```python
from build123d import *

# Parameters (mm, degrees)
SKETCH_1_W      = 68.5
SKETCH_1_H      = 36.5
SKETCH_1_W_2    = 56.5
SKETCH_1_H_2    = 24.5
EXTRUDE_1_DEPTH = 1
FILLET_1_R      = 3


with BuildPart() as part:
    # 草图1 → 凸台-拉伸1 (new body)
    with BuildSketch(Plane(origin=(0, 0, 0), x_dir=(1, 0, 0), z_dir=(0, 1, 0))):
        with Locations((-124.87745098, 48.691176471)):
            Rectangle(SKETCH_1_W, SKETCH_1_H)
        with Locations((-124.87745098, 48.691176471)):
            Rectangle(SKETCH_1_W_2, SKETCH_1_H_2, mode=Mode.SUBTRACT)
    extrude(amount=EXTRUDE_1_DEPTH)

    # 圆角1
    fillet_1_edges = [part.edges().sort_by_distance(p)[0] for p in [
        (-159.12745098, 0.5, -66.941176471),
        (-90.62745098, 0.5, -66.941176471),
        (-90.62745098, 0.5, -30.441176471),
        (-159.12745098, 0.5, -30.441176471),
    ]]
    fillet(fillet_1_edges, radius=FILLET_1_R)


solid = part.part
```
For this review, take the finished solid that the model builds, in its own axes (mm). Give positions to 0.01 mm unless a question says otherwise; leave off trailing zeros. Write each loop counter-clockwise with the first axis right and the second up, starting at its lowest first coordinate (ties: lowest second). Pieces come first, ordered by that corner, then holes. Notation, with made-up numbers: M -38.5,18 L 12.5,18 A32 cw 12.5,52 Z; hole C -13.5,12 d9. An arc over 180 degrees is marked long. Answer as a JSON object with one key per item and string values. Group by question number.
Item 1: Consider section A-A on z = -60. Write out the cut boundary in (x, y), plus the area to 3 significant figures.
Item 2: Consider section C-C on y = 0.65. Write out the cut boundary in (x, z), plus the area to 3 significant figures.
Item 3: For probe 1 along Z at (x, y) = (-140, 0.1); probe 2 along X at (y, z) = (0.3, -43.5); probe 3 along Z at (x, y) = (-93.5, 0.3), list the stretches that pass through material, from the lowest coordinate up. Write a range as [from, to].
Item 4: Consider section B-B on x = -131. Write out the cut boundary in (y, z).
Check result:
{
 "1": {"outline": "M -159.13,0 L -153.13,0 L -153.13,1 L -159.13,1 Z; M -96.63,0 L -90.63,0 L -90.63,1 L -96.63,1 Z", "area": "12.0 mm^2"},
 "2": {"outline": "M -159.13,-63.94 A3 ccw -156.13,-66.94 L -93.63,-66.94 A3 ccw -90.63,-63.94 L -90.63,-33.44 A3 ccw -93.63,-30.44 L -156.13,-30.44 A3 ccw -159.13,-33.44 Z; hole M -153.13,-60.94 L -96.63,-60.94 L -96.63,-36.44 L -153.13,-36.44 Z", "area": "1,110 mm^2"},
 "3": {"probe 1": "z = [-66.94, -60.94], [-36.44, -30.44]", "probe 2": "x = [-159.13, -153.13], [-96.63, -90.63]", "probe 3": "z = [-66.94, -30.44]"},
 "4": {"outline": "M 0,-66.94 L 1,-66.94 L 1,-60.94 L 0,-60.94 Z; M 0,-36.44 L 1,-36.44 L 1,-30.44 L 0,-30.44 Z"}
}
